from build123d import *

# Parameters (mm, degrees)
ESQUISSE1_W             = 1126
ESQUISSE1_H             = 297
ESQUISSE1_R             = 1.5
BOSS_EXTRU_1_DEPTH      = 12
ESQUISSE2_W             = 15
ESQUISSE2_H             = 678.559774038
ESQUISSE2_H_2           = 656.681006804
ENL_V_MAT_EXTRU_1_DEPTH = 4


with BuildPart() as part:
    # Esquisse1 → Boss.-Extru.1 (new body)
    with BuildSketch(Plane.XY):
        Rectangle(ESQUISSE1_W, ESQUISSE1_H)
        with Locations((105.5, 98.5)):
            Circle(ESQUISSE1_R, mode=Mode.SUBTRACT)
        with Locations((105.5, -98.5)):
            Circle(ESQUISSE1_R, mode=Mode.SUBTRACT)
        with Locations((-355.5, 98.5)):
            Circle(ESQUISSE1_R, mode=Mode.SUBTRACT)
        with Locations((-355.5, -98.5)):
            Circle(ESQUISSE1_R, mode=Mode.SUBTRACT)
        with BuildLine():
            Line((255.5, 96.5), (413, 96.5))
            ThreePointArc((413, 96.5), (513, -3.5), (413, -103.5))
            Line((413, -103.5), (255.5, -103.5))
            ThreePointArc((255.5, -103.5), (155.5, -3.5), (255.5, 96.5))
        make_face(mode=Mode.SUBTRACT)
    extrude(amount=BOSS_EXTRU_1_DEPTH)

    # Esquisse2 → Enlèv. mat.-Extru.1 (cut)
    with BuildSketch(Plane(origin=(0, 0, 0), x_dir=(-1, 0, 0), z_dir=(0, 0, -1))):
        with Locations((-105.5, 98.5)):
            Rectangle(ESQUISSE2_W, ESQUISSE2_H)
        with Locations((355.5, 98.5)):
            Rectangle(ESQUISSE2_W, ESQUISSE2_H_2)
    extrude(amount=-ENL_V_MAT_EXTRU_1_DEPTH, mode=Mode.SUBTRACT)


solid = part.part
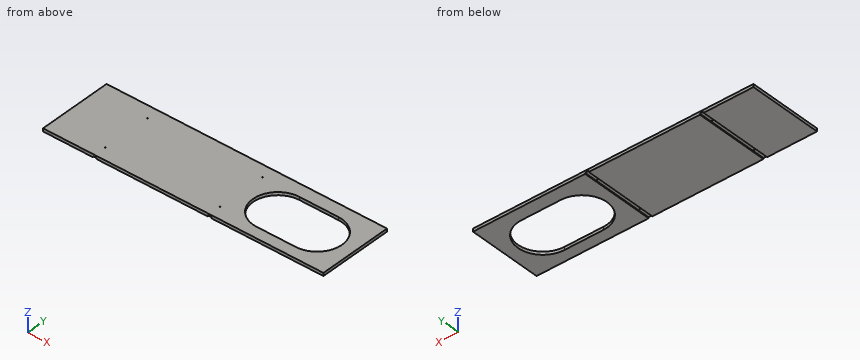
The model under review builds one solid part; all positions refer to its coordinate system, in mm. Give positions to 0.01 mm unless a question says otherwise; leave off trailing zeros. Order: outer loops, then holes, each group sorted by start corner. A loop starts at its lowest first (then second) coordinate and runs counter-clockwise, first axis right, second up. Notation, with made-up numbers: (61, 14) -> (96, 14) arc R21 cw to (96, 35) -> close; hole circle Ø5 at (9.25, -19.75). An arc over 180 degrees is marked (long way). Write item = value, one per line. Start each with the question number.
(1) For L1, parallel to Y at x = 105.5, z = 10; L2, parallel to X at y = 98.5, z = 7; L3, parallel to X at y = -10, z = 0.5, list the stretches that pass through material, from the lowest coordinate up. Write a range as from..to.
(2) For pin 1 Ø2.5 at (x, y) = (105.5, -98.5) entering from +Z; pin 2 Ø4 at (x, y) = (-355.5, -98.5) entering from -Z, all flat-tipped, find the tip position at first contact; note any pin that passes through.
(3) Take a section at A-A (y = -3.5). Write out the cut boundary in (x, z), plus the area to 3 significant figures.
(4) Take a section at B-B (z = 6.75). Write out the cut boundary in (x, y).
Returned:
q1.L1 = -148.5..-100, -97..97, 100..148.5
q1.L2 = -563..-357, -354..104, 107..563
q1.L3 = -563..-363, -348..98, 113..155.71, 512.79..563
q2.pin_1 = through
q2.pin_2 = 4
q3.outline = (-563, 0) -> (-363, 0) -> (-363, 4) -> (-348, 4) -> (-348, 0) -> (98, 0) -> (98, 4) -> (113, 4) -> (113, 0) -> (155.5, 0) -> (155.5, 12) -> (-563, 12) -> close; (513, 0) -> (563, 0) -> (563, 12) -> (513, 12) -> close
q3.area = 9,100 mm²
q4.outline = (-563, -148.5) -> (563, -148.5) -> (563, 148.5) -> (-563, 148.5) -> close; hole circle Ø3 at (-355.5, -98.5); hole circle Ø3 at (-355.5, 98.5); hole circle Ø3 at (105.5, -98.5); hole circle Ø3 at (105.5, 98.5); hole (255.5, -103.5) -> (413, -103.5) arc R100 ccw to (413, 96.5) -> (255.5, 96.5) arc R100 ccw to start
